Read the model definition and answer for the solid it produces. Units are mm, in the model's axes. Face numbers are marked on the shaded views. A direction names the side the tool comes from. Coordinates: 2 decimals unless noted, no trailing zeros. Write each loop counter-clockwise with the first axis right and the second up, starting at its lowest first coordinate (ties: lowest second). Pieces come first, ordered by that corner, then holes. Notation, with made-up numbers: (39.25, 78.25) - (86.25, 78.25) arc R24 ccw to (86.25, 104.25) - close; hole circle Ø1 at (-12, -5.75). An arc over 180 degrees is marked (long way). Use a Markdown table: item, result.
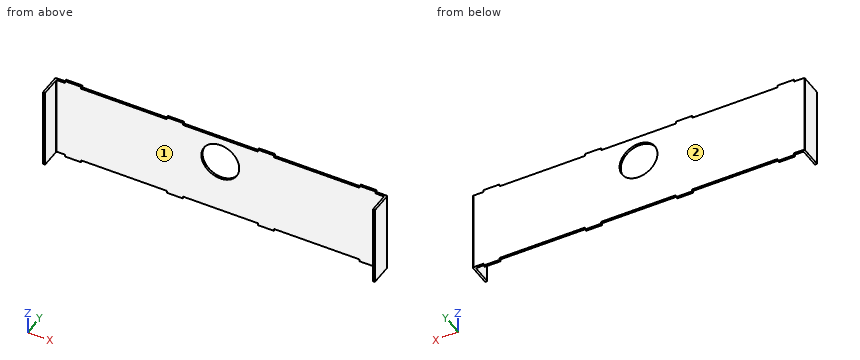
from build123d import *

# Parameters (mm, degrees)
SKETCH_1_R      = 17.7
EXTRUDE_1_DEPTH = 2
SKETCH_2_W      = 2
SKETCH_2_H      = 76
EXTRUDE_2_DEPTH = 19
FILLET_1_R      = 1


with BuildPart() as part:
    # 草图1 → 凸台-拉伸1 (new body)
    with BuildSketch(Plane(origin=(0, 0, 0), x_dir=(1, 0, 0), z_dir=(0, 1, 0))):
        Polygon((-155, -38), (-145, -38), (-145, -40), (-130, -40), (-130, -38), (-50, -38), (-50, -40), (-35, -40), (-35, -38), (35, -38), (35, -40), (50, -40), (50, -38), (130, -38), (130, -40), (145, -40), (145, -38), (155, -38), (155, 38), (145, 38), (145, 40), (130, 40), (130, 38), (50, 38), (50, 40), (35, 40), (35, 38), (-35, 38), (-35, 40), (-50, 40), (-50, 38), (-130, 38), (-130, 40), (-145, 40), (-145, 38), (-155, 38), align=None)
        with Locations(Location((0, -13, 0), (0, 0, 270))):
            Circle(SKETCH_1_R, mode=Mode.SUBTRACT)
    extrude(amount=EXTRUDE_1_DEPTH)

    # 草图2 → 凸台-拉伸2 (add)
    with BuildSketch(Plane.XZ):
        with Locations((154, 0)):
            Rectangle(SKETCH_2_W, SKETCH_2_H)
    extrude_2 = extrude(amount=EXTRUDE_2_DEPTH)

    # 镜向1: 凸台-拉伸2 across plane
    add(extrude_2.mirror(Plane(origin=(0, 0, 0), x_dir=(0, 0, 1), z_dir=(1, 0, 0))))

    # 圆角1
    fillet_1_edges = [part.edges().sort_by_distance(p)[0] for p in [
        (153, 0, 0),
        (155, 2, 0),
        (-153, 0, 0),
        (-155, 2, 0),
    ]]
    fillet(fillet_1_edges, radius=FILLET_1_R)


solid = part.part
(1) A cutting plane is placed at D-D, the plane z = -13.5. Write down the section's boundary in (x, y), and give its area (3 significant figures).
Report:
| item | result |
|---|---|
| outline | (-155, -19) - (-153, -19) - (-153, -1) arc R1 cw to (-152, 0) - (152, 0) arc R1 cw to (153, -1) - (153, -19) - (155, -19) - (155, 1) arc R1 ccw to (154, 2) - (-154, 2) arc R1 ccw to (-155, 1) - close |
| area | 696 mm² |
(2) For the marked faces 1 and 2, determine the directions among +Z, -Z, +X, -X, +Y, -Y from which every point of the face is accessible in a straight line to the end or side of a thin tool.
Report:
| item | result |
|---|---|
| face 1 | +Z, -Z, -Y |
| face 2 | +Z, -Z, +X, -X, +Y |
(3) A cutting plane is placed at C-C, the plane x = 0. Write down the section's boundary in (y, z), and give its area (3 significant figures).
Report:
| item | result |
|---|---|
| outline | (0, -38) - (2, -38) - (2, -4.7) - (0, -4.7) - close; (0, 30.7) - (2, 30.7) - (2, 38) - (0, 38) - close |
| area | 81.2 mm² |
(4) A cutting plane is placed at B-B, the plane z = 13. Write down the section's boundary in (x, y), and give its area (3 significant figures).
Report:
| item | result |
|---|---|
| outline | (-155, -19) - (-153, -19) - (-153, -1) arc R1 cw to (-152, 0) - (-17.7, 0) - (-17.7, 2) - (-154, 2) arc R1 ccw to (-155, 1) - close; (17.7, 0) - (152, 0) arc R1 cw to (153, -1) - (153, -19) - (155, -19) - (155, 1) arc R1 ccw to (154, 2) - (17.7, 2) - close |
| area | 625 mm² |
(5) Straight lines are drawn through the part: L1, parallel to X at y = -7.25, z = 33.5; L2, parallel to X at y = 0.85, z = 13; L3, parallel to Y at x = -3.5, z = -14. For each, find the intervals that lie inside material, in ascending order.
Report:
| item | result |
|---|---|
| L1 | x = -155 to -153, 153 to 155 |
| L2 | x = -155 to -17.7, 17.7 to 155 |
| L3 | y = 0 to 2 |
(6) Each of these flat-tipped pins is pushed along its axis until it touches: P1, Ø1.6, axis at y = 1, z = -39.5, coming from the -X side; P2, Ø24, axis at x = -31.5, z = -2.5, coming from the -Y side; P3, Ø5, axis at x = 111, y = -4, coming from the -Z side; P4, Ø2, axis at x = 99.5, y = 0.5, coming from the -Z side. Where does it stop, or does it pass through?
Report:
| item | result |
|---|---|
| P1 | stops at x = -145 |
| P2 | stops at y = 0 |
| P3 | passes through |
| P4 | stops at z = -38 |
(7) A cutting plane is placed at A-A, the plane y = -7.5. Write down the section's boundary in (x, z).
Report:
| item | result |
|---|---|
| outline | (-155, -38) - (-153, -38) - (-153, 38) - (-155, 38) - close; (153, -38) - (155, -38) - (155, 38) - (153, 38) - close |
